from build123d import *

# Parameters (mm, degrees)
SKETCH1_W               = 889
SKETCH1_H               = 31.75
EXTRUDE1_DEPTH          = 28.575
EXTRUDE2_REACH          = 891
SKETCH2_W               = 25.4
SKETCH2_H               = 25.4
HOLE1_D                 = 6.35
HOLE1_DEPTH             = 3.175
LPATTERN1_COUNT         = 35
LPATTERN1_PITCH         = 25.4
HOLE2_D                 = 9.652
HOLE2_DEPTH             = 3.175
LPATTERN2_COUNT         = 12
LPATTERN2_PITCH         = 25.4
HOLE3_D                 = 9.652
HOLE3_DEPTH             = 3.175
HOLE4_D                 = 9.652
HOLE4_DEPTH             = 3.175
LPATTERN3_COUNT         = 12
LPATTERN3_PITCH         = 25.4
HOLE5_D                 = 3.175
HOLE5_DEPTH             = 3.175
HOLE6_D                 = 6.35
HOLE6_DEPTH             = 3.175
LPATTERN4_COUNT         = 35
LPATTERN4_PITCH         = 25.4
FILLET1_R               = 3.175
FILLET2_R               = 3.175
FILLET3_R               = 6.35
FILLET4_R               = 6.35
SKETCH15_W              = 739
SKETCH15_H              = 22.225
SKETCH15_R              = 3.175
CUT_EXTRUDE4_DEPTH      = 77
CUT_EXTRUDE4_DEPTH_BACK = 92


with BuildPart() as part:
    # Sketch1 → Extrude1 (new body)
    with BuildSketch(Plane.XY.offset(3.175)):
        with Locations((428.480011997, 8.672957166)):
            Rectangle(SKETCH1_W, SKETCH1_H)
    extrude(amount=-EXTRUDE1_DEPTH)

    # Sketch2 → Extrude2 (cut, up to next)
    with BuildSketch(Plane.ZY.offset(16.019988003), mode=Mode.PRIVATE) as extrude2_sk1:
        with Locations((-12.7, 8.672957166)):
            Rectangle(SKETCH2_W, SKETCH2_H)
    extrude2_tool1 = extrude(extrude2_sk1.sketch, amount=-EXTRUDE2_REACH, mode=Mode.PRIVATE) & part.part
    add(extrude2_tool1.solids().sort_by_distance((-16.019988, 8.672957, -12.7))[0], mode=Mode.SUBTRACT)

    # Hole1
    with Locations(Plane(origin=(0, 24.547957166, 0), x_dir=(-1, 0, 0), z_dir=(0, 1, 0))):
        with Locations((3.319988003, -12.7)):
            hole1 = Hole(HOLE1_D / 2, depth=HOLE1_DEPTH)

    # LPattern1: Hole1 ×35
    with Locations(*[(i * LPATTERN1_PITCH, 0, 0) for i in range(1, LPATTERN1_COUNT)]):
        add(hole1, mode=Mode.SUBTRACT)

    # Hole2
    with Locations(Plane.XY.offset(3.175)):
        with Locations((66.530011997, 10.577957166)):
            hole2 = Hole(HOLE2_D / 2, depth=HOLE2_DEPTH)

    # LPattern2: Hole2 ×12, 8 skipped
    with Locations(*[(i * LPATTERN2_PITCH, 0, 0) for i in range(1, LPATTERN2_COUNT) if i not in (2, 3, 4, 5, 6, 7, 8, 9)]):
        add(hole2, mode=Mode.SUBTRACT)

    # Hole3
    with Locations(Plane.XY.offset(3.175)):
        with Locations((428.480011997, 6.767957166)):
            Hole(HOLE3_D / 2, depth=HOLE3_DEPTH)

    # Hole4
    with Locations(Plane.XY.offset(3.175)):
        with Locations((511.030011997, 10.577957166)):
            hole4 = Hole(HOLE4_D / 2, depth=HOLE4_DEPTH)

    # LPattern3: Hole4 ×12, 8 skipped
    with Locations(*[(i * LPATTERN3_PITCH, 0, 0) for i in range(1, LPATTERN3_COUNT) if i not in (2, 3, 4, 5, 6, 7, 8, 9)]):
        add(hole4, mode=Mode.SUBTRACT)

    # Hole5
    with Locations(Plane.XY.offset(3.175)):
        with Locations((669.780011997, 8.672957166)):
            Hole(HOLE5_D / 2, depth=HOLE5_DEPTH)

    # Hole6
    with Locations(Plane(origin=(0, -4.027042834, 0), x_dir=(-1, 0, 0), z_dir=(0, 1, 0))):
        with Locations((3.319988003, -12.7)):
            hole6 = Hole(HOLE6_D / 2, depth=HOLE6_DEPTH)

    # LPattern4: Hole6 ×35
    with Locations(*[(i * LPATTERN4_PITCH, 0, 0) for i in range(1, LPATTERN4_COUNT)]):
        add(hole6, mode=Mode.SUBTRACT)

    # Fillet1
    fillet1_edges = [part.edges().sort_by_distance(p)[0] for p in [
        (428.480011997, 21.372957166, 0),
    ]]
    fillet(fillet1_edges, radius=FILLET1_R)

    # Fillet2
    fillet2_edges = [part.edges().sort_by_distance(p)[0] for p in [
        (428.480011997, -4.027042834, 0),
    ]]
    fillet(fillet2_edges, radius=FILLET2_R)

    # Fillet3
    fillet3_edges = [part.edges().sort_by_distance(p)[0] for p in [
        (428.480011997, -7.202042834, 3.175),
    ]]
    fillet(fillet3_edges, radius=FILLET3_R)

    # Fillet4
    fillet4_edges = [part.edges().sort_by_distance(p)[0] for p in [
        (428.480011997, 24.547957166, 3.175),
    ]]
    fillet(fillet4_edges, radius=FILLET4_R)

    # Sketch15 → Cut-Extrude4 (cut, two sides)
    with BuildSketch(Plane(origin=(0, 24.547957166, 0), x_dir=(1, 0, 0), z_dir=(0, 1, 0))) as cut_extrude4_sk:
        Polygon((-16.019988003, 3.175), (-16.019988003, 25.4), (-76.590899014, 25.4), (-76.590899014, -29.102378411), (722.980011997, -29.102378411), (722.980011997, 3.175), align=None)
        with Locations((353.480011997, 14.2875)):
            Rectangle(SKETCH15_W, SKETCH15_H)
        with Locations((-3.319988003, 12.7)):
            Circle(SKETCH15_R, mode=Mode.SUBTRACT)
        with Locations((47.480011997, 12.7)):
            Circle(SKETCH15_R, mode=Mode.SUBTRACT)
        with Locations((98.280011997, 12.7)):
            Circle(SKETCH15_R, mode=Mode.SUBTRACT)
        with Locations((149.080011997, 12.7)):
            Circle(SKETCH15_R, mode=Mode.SUBTRACT)
        with Locations((199.880011997, 12.7)):
            Circle(SKETCH15_R, mode=Mode.SUBTRACT)
        with Locations((250.680011997, 12.7)):
            Circle(SKETCH15_R, mode=Mode.SUBTRACT)
        with Locations((301.480011997, 12.7)):
            Circle(SKETCH15_R, mode=Mode.SUBTRACT)
        with Locations((326.880011997, 12.7)):
            Circle(SKETCH15_R, mode=Mode.SUBTRACT)
        with Locations((352.280011997, 12.7)):
            Circle(SKETCH15_R, mode=Mode.SUBTRACT)
        with Locations((377.680011997, 12.7)):
            Circle(SKETCH15_R, mode=Mode.SUBTRACT)
        with Locations((403.080011997, 12.7)):
            Circle(SKETCH15_R, mode=Mode.SUBTRACT)
        with Locations((428.480011997, 12.7)):
            Circle(SKETCH15_R, mode=Mode.SUBTRACT)
        with Locations((453.880011997, 12.7)):
            Circle(SKETCH15_R, mode=Mode.SUBTRACT)
        with Locations((479.280011997, 12.7)):
            Circle(SKETCH15_R, mode=Mode.SUBTRACT)
        with Locations((504.680011997, 12.7)):
            Circle(SKETCH15_R, mode=Mode.SUBTRACT)
        with Locations((530.080011997, 12.7)):
            Circle(SKETCH15_R, mode=Mode.SUBTRACT)
        with Locations((555.480011997, 12.7)):
            Circle(SKETCH15_R, mode=Mode.SUBTRACT)
        with Locations((580.880011997, 12.7)):
            Circle(SKETCH15_R, mode=Mode.SUBTRACT)
        with Locations((606.280011997, 12.7)):
            Circle(SKETCH15_R, mode=Mode.SUBTRACT)
        with Locations((631.680011997, 12.7)):
            Circle(SKETCH15_R, mode=Mode.SUBTRACT)
        with Locations((657.080011997, 12.7)):
            Circle(SKETCH15_R, mode=Mode.SUBTRACT)
        with Locations((682.480011997, 12.7)):
            Circle(SKETCH15_R, mode=Mode.SUBTRACT)
        with Locations((707.880011997, 12.7)):
            Circle(SKETCH15_R, mode=Mode.SUBTRACT)
    extrude(amount=CUT_EXTRUDE4_DEPTH, mode=Mode.SUBTRACT)
    extrude(cut_extrude4_sk.sketch, amount=-CUT_EXTRUDE4_DEPTH_BACK, mode=Mode.SUBTRACT)


solid = part.part
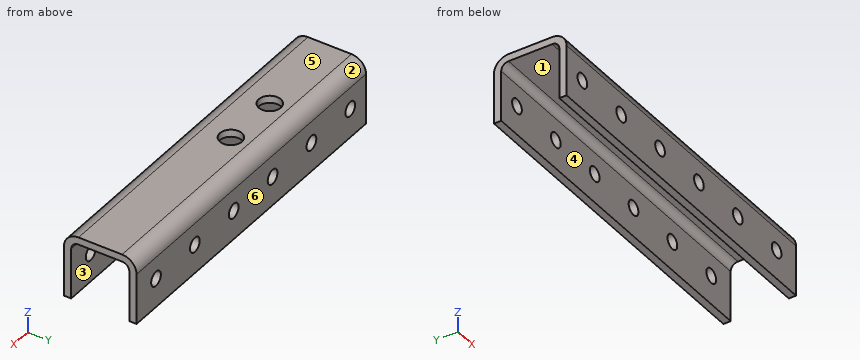
Part model, mm, in its own coordinate system. Face numbers are marked on the shaded views. A direction names the side the tool comes from. Coordinates: 2 decimals unless noted, no trailing zeros. Order: outer loops, then holes, each group sorted by start corner. A loop starts at its lowest first (then second) coordinate and runs counter-clockwise, first axis right, second up.
(1) Tool access for the marked faces 1 and 2: list every direction of +Z, -Z, +X, -X, +Y, -Y with a clear straight run to the whole face (end or side of a thin tool).
Check sheet entries:
face 1: -Z, +X, -X
face 2: +Z, +X, -X, +Y
(2) Pin check, flat tips, straight feed: pin 1 Ø3 at (x, y) = (836.5, 15) entering from -Z; pin 2 Ø1 at (x, y) = (814, -4) entering from +Z. Stop position of each tip, or through.
Check sheet entries:
pin 1: stops at z = 0
pin 2: stops at z = 2.6
(3) Slice it at C-C, the plane y = 4. Write the cut outline in (x, z) (3 decimals), and give its area (3 significant figures).
Check sheet entries:
outline: (722.98, 0) - (872.98, 0) - (872.98, 3.175) - (722.98, 3.175) - close
area: 476 mm2
(4) Probe L1, parallel to Y at x = 757, z = -18; L2, parallel to Z at x = 812.5, y = 1.5 (3 decimals); L3, parallel to Y at x = 822, z = -2. List the from-to ranges inside material, lowest first.
Check sheet entries:
L1: y = -7.2 to -4.03, 21.37 to 24.55
L2: z = 0 to 3.175
L3: y = -7.09 to -3.8, 21.15 to 24.44
(5) Slice it at B-B, the plane x = 793.5. Write the cut outline in (y, z) (3 decimals), and give its area (3 significant figures).
Check sheet entries:
outline: (-7.202, -25.4) - (-4.027, -25.4) - (-4.027, -3.175) arc R3.175 cw to (-0.852, 0) - (6.854, 0) - (6.854, 3.175) - (-0.852, 3.175) arc R6.35 ccw to (-7.202, -3.175) - close; (14.302, 0) - (18.198, 0) arc R3.175 cw to (21.373, -3.175) - (21.373, -25.4) - (24.548, -25.4) - (24.548, -3.175) arc R6.35 ccw to (18.198, 3.175) - (14.302, 3.175) - close
area: 225 mm2
(6) Slice it at A-A, the plane z = -8.25. Write the cut outline in (x, y), and give its area (4 significant figures).
Check sheet entries:
outline: (722.98, -7.2) - (872.98, -7.2) - (872.98, -4.03) - (722.98, -4.03) - close; (722.98, 21.37) - (872.98, 21.37) - (872.98, 24.55) - (722.98, 24.55) - close
area: 952.5 mm2
(7) Pull direction Y, two halves, no side cores. Call the marked faces 3, 4, 5 and 6: pulls with the +Y half, pulls with the -Y half, needs draft (parallel to the pull), parting line crosses it, or undercut.
Check sheet entries:
face 3: undercut
face 4: undercut
face 5: needs draft
face 6: pulls with the +Y half
